```python
from build123d import *

# Parameters (mm, degrees)
CUT_EXTRUDE1_DEPTH  = 50
FILLET1_R           = 5
SKETCH4_R           = 7.5
CUT_EXTRUDE2_DEPTH  = 3
SKETCH6_R           = 5
CUT_EXTRUDE3_DEPTH  = 21
SKETCH7_R           = 6
BOSS_EXTRUDE1_DEPTH = 62
CUT_EXTRUDE4_START  = -100
SKETCH8_R           = 5
CUT_EXTRUDE4_DEPTH  = 100


with BuildPart() as part:
    # Sketch1 → Revolve1 (revolve)
    with BuildSketch(Plane.XY, mode=Mode.PRIVATE) as revolve1_sk:
        with BuildLine():
            Line((35, 65), (35, 60))
            Line((35, 60), (32.5, 60))
            Line((32.5, 60), (32.5, 57.5))
            Line((32.5, 57.5), (35, 57.5))
            Line((35, 57.5), (35, 55))
            Line((35, 55), (32.5, 55))
            Line((32.5, 55), (32.5, 52.5))
            Line((32.5, 52.5), (35, 52.5))
            Line((35, 52.5), (35, 50))
            Line((35, 50), (32.5, 50))
            Line((32.5, 50), (32.5, 47.5))
            Line((32.5, 47.5), (35, 47.5))
            Line((35, 47.5), (35, 0))
            Line((35, 0), (29, 0))
            Line((29, 0), (29, 41.5))
            Line((29, 41.5), (26.5, 41.5))
            Line((26.5, 41.5), (26.5, 51.25))
            Line((26.5, 51.25), (26.5, 56.25))
            Line((26.5, 56.25), (26.5, 60.153370447))
            Line((26.5, 60.153370447), (0, 63.939084733))
            Line((0, 63.939084733), (0, 70))
            ThreePointArc((0, 70), (17.762839264, 69.339874847), (35, 65))
        make_face()
    revolve(revolve1_sk.sketch.rotate(Axis((0, 0, 0), (0, 1, 0)), 90), axis=Axis((0, 0, 0), (0, 1, 0)))

    # Sketch2 → Cut-Extrude1 (cut, symmetric)
    with BuildSketch(Plane.XY):
        Polygon((-10, 9.214548861), (10, 9.214548861), (14.296814701, 0), (14.296814701, -4.920765988), (0.577416947, -4.920765988), (-8.331342859, -4.920765988), (-14.2968147, 0), align=None)
    extrude(amount=CUT_EXTRUDE1_DEPTH, both=True, mode=Mode.SUBTRACT)

    # Fillet1
    fillet1_edges = [part.edges().sort_by_distance(p)[0] for p in [
        (14.296814701, 0, -28.588901432),
        (14.296814701, 0, 28.588901432),
        (10, 9.214548861, 30.38116742),
        (10, 9.214548861, -30.38116742),
        (-14.2968147, 0, 28.588901432),
        (-14.2968147, 0, -28.588901432),
        (-10, 9.214548861, 30.38116742),
        (-10, 9.214548861, -30.38116742),
    ]]
    fillet(fillet1_edges, radius=FILLET1_R)

    # Sketch4 → Cut-Extrude2 (cut)
    with BuildSketch(Plane.ZY.offset(35)):
        with Locations((0, 23.312730986)):
            Circle(SKETCH4_R)
    cut_extrude2 = extrude(amount=-CUT_EXTRUDE2_DEPTH, mode=Mode.SUBTRACT)

    # Sketch6 → Cut-Extrude3 (cut)
    with BuildSketch(Plane.ZY.offset(32)):
        with Locations((0, 23.312730986)):
            Circle(SKETCH6_R)
    cut_extrude3 = extrude(amount=-CUT_EXTRUDE3_DEPTH, mode=Mode.SUBTRACT)

    # Mirror1: Cut-Extrude2, Cut-Extrude3 across plane
    add(cut_extrude2.mirror(Plane(origin=(0, 0, 0), x_dir=(0, 0, 1), z_dir=(1, 0, 0))), mode=Mode.SUBTRACT)
    add(cut_extrude3.mirror(Plane(origin=(0, 0, 0), x_dir=(0, 0, 1), z_dir=(1, 0, 0))), mode=Mode.SUBTRACT)

    # Sketch7 → Boss-Extrude1 (add)
    with BuildSketch(Plane(origin=(32, 0, 0), x_dir=(0, 0, -1), z_dir=(1, 0, 0))):
        with Locations((0, 23.312730986)):
            Circle(SKETCH7_R)
    extrude(amount=-BOSS_EXTRUDE1_DEPTH)

    # Sketch8 → Cut-Extrude4 (cut)
    with BuildSketch(Plane(origin=(32, 0, 0), x_dir=(0, 0, -1), z_dir=(1, 0, 0)).offset(CUT_EXTRUDE4_START)):
        with Locations(Location((0, 23.312730986, 0), (0, 0, 180))):
            Circle(SKETCH8_R)
    extrude(amount=CUT_EXTRUDE4_DEPTH, mode=Mode.SUBTRACT)


solid = part.part
```
Geometry: final body of the model. Coordinates: model frame, mm. A direction names the side the tool comes from. Coordinates: 2 decimals unless noted, no trailing zeros. Order: outer loops, then holes, each group sorted by start corner. A loop starts at its lowest first (then second) coordinate and runs counter-clockwise, first axis right, second up. Notation, with made-up numbers: (13, -21.5) - (19, -21.5) arc R17 ccw to (19, -10.5) - close; hole circle Ø5 at (84.25, 7). An arc over 180 degrees is marked (long way). Return JSON: item names as keys, results as strings. Group by question number.
1. Pin query (flat end, axial travel): pin 1 (13 mm diameter, centred on y = 23.31, z = 0, fed in from -X); pin 2 (3 mm diameter, centred on y = 51, z = -22, fed in from +X); pin 3 (1 mm diameter, centred on x = -16.5, y = 19.5, fed in from -Z). Return the tip coordinate at first contact, or that it passes through.
2. Pull-direction query (X, two-part tool) for faces 1 (the face through (-9.47, 8.45, -30.46)), 2 (the face through (-9.76, 48.73, -31)), 3 (the face through (23.2, 55, -23.2)); classes: pulls with the +X half, pulls with the -X half, needs draft (parallel to the pull), parting line crosses it, or undercut.
3. Material intervals for line 1 along Z through (x, y) = (-0.5, 29.5); line 2 along X through (y, z) = (36, 17.5), sorted ascending. Write a range as [from, to].
4. Cut plane B-B (y = 59). Output: boundary loops of the cut face in (x, z), plus the area to 3 significant figures.
5. Cut plane C-C (x = 4). Count the separate pieces of the cut face and the enclosed holes in it, plus the area to 3 significant figures.
6. Cut plane A-A (y = 19.5). Output: boundary loops of the cut face in (x, z).
7. Set-up query: faces 4 (the face through (-32, 22, 5)), 5 (the face through (30, 0, 0)), 6 (the face through (23.2, 47.5, 23.2)), 7 (the face through (14.762, 0.805, 27.761)). Return all of +Z, -Z, +X, -X, +Y, -Y with unobstructed straight access to the full face (end or side cutting, diameter ignored); none if empty.
Resolved:
{
 "1": {"pin 1": "stops at x = -32", "pin 2": "stops at x = 28.37", "pin 3": "stops at z = -31.13"},
 "2": {"face 1": "undercut", "face 2": "parting line crosses it", "face 3": "needs draft"},
 "3": {"line 1": "z = [-35, -29], [29, 35]", "line 2": "x = [-30.31, -23.12], [23.12, 30.31]"},
 "4": {"outline": "circle Ø65 at (0, 0); hole circle Ø53 at (0, 0)", "area": "1,110 mm²"},
 "5": {"separate pieces": "2", "enclosed holes": "1", "area": "1,210 mm²"},
 "6": {"outline": "(-34.4, -6.46) arc R35 ccw to (34.4, -6.46) - (32, -6.46) - (32, -3.23) - (-32, -3.23) - (-32, -6.46) - close; (-34.4, 6.46) - (-32, 6.46) - (-32, 3.23) - (32, 3.23) - (32, 6.46) - (34.4, 6.46) arc R35 ccw to start; hole (-28.63, -4.63) arc R29 ccw to (28.63, -4.63) - close; hole (-28.63, 4.63) - (28.63, 4.63) arc R29 ccw to start"},
 "7": {"face 4": "-X", "face 5": "+Z, -Z, +X, -X, -Y", "face 6": "none", "face 7": "+Z, -Z, -Y"}
}
